```python
from build123d import *

# Parameters (mm, degrees)
SKETCH2_R              = 24.13
SKETCH2_R_2            = 20.447
BASE_DEPTH             = 304.8
SNAP_RING_GROOVE_START = -6.35
SKETCH3_R              = 21.9075
SKETCH3_R_2            = 20.447
SNAP_RING_GROOVE_DEPTH = 1.7272


with BuildPart() as part:
    # Sketch2 → base (new body)
    with BuildSketch(Plane(origin=(0, 0, 0), x_dir=(0, 1, 0), z_dir=(0, 0, 1))):
        with Locations(Location((0, 0, 0), (0, 0, 90))):
            Circle(SKETCH2_R)
        with Locations(Location((0, 0, 0), (0, 0, 90))):
            Circle(SKETCH2_R_2, mode=Mode.SUBTRACT)
    extrude(amount=BASE_DEPTH)

    # Sketch3 → snap_ring_groove (cut)
    with BuildSketch(Plane(origin=(0, 0, 0), x_dir=(1, 0, 0), z_dir=(0, 0, -1)).offset(SNAP_RING_GROOVE_START)):
        with Locations(Location((0, 0, 0), (0, 0, 180))):
            Circle(SKETCH3_R)
        with Locations(Location((0, 0, 0), (0, 0, 180))):
            Circle(SKETCH3_R_2, mode=Mode.SUBTRACT)
    extrude(amount=-SNAP_RING_GROOVE_DEPTH, mode=Mode.SUBTRACT)


solid = part.part
```
Part model, mm, in its own coordinate system. A direction names the side the tool comes from. Coordinates: 2 decimals unless noted, no trailing zeros. Write each loop counter-clockwise with the first axis right and the second up, starting at its lowest first coordinate (ties: lowest second). Pieces come first, ordered by that corner, then holes.
Item 1: Slice it at A-A (x = 0). Write the cut outline in (y, z).
Item 2: Pin check, flat tips, straight feed: pin 1 (10 mm diameter, centred on x = 0, z = 223.5, fed in from +Y); pin 2 (24.5 mm diameter, centred on x = 0, y = 0, fed in from -Z); pin 3 (3 mm diameter, centred on x = 13, z = 257, fed in from -Y); pin 4 (12 mm diameter, centred on y = 10, z = 267, fed in from -X). Stop position of each tip, or through.
Item 3: Probe line 1 (Z direction, x = 4, y = 20.5); line 2 (Y direction, x = 0, z = 7.5); line 3 (Y direction, x = 0, z = 90.5). List the from-to ranges inside material, lowest first.
Item 4: Slice it at C-C (z = 184.5). Write the cut outline in (x, y), and give its area (3 significant figures).
Item 5: Which spindle directions (+Z, -Z, +X, -X, +Y, -Y) get a long thin tool onto all of the face, cutting with end or side? Do faces 1 (the face through (4.749, -21.387, 7.202)), 2 (the face through (20, -5, 0)). Say none if no direction does.
Item 6: Mould opens along Z. For faces 3 (the face through (20, -5, 304.8)), 4 (the face through (16.226, 12.442, 154.362)), 5 (the face through (-15, -15, 8.077)), 6 (the face through (-15, -15, 6.35)) say: released by +Z, released by -Z, zero draft, split by the parting line, or undercut.
Results found:
1. outline: (-24.13, 0) - (-20.45, 0) - (-20.45, 6.35) - (-21.91, 6.35) - (-21.91, 8.08) - (-20.45, 8.08) - (-20.45, 304.8) - (-24.13, 304.8) - close; (20.45, 0) - (24.13, 0) - (24.13, 304.8) - (20.45, 304.8) - (20.45, 8.08) - (21.91, 8.08) - (21.91, 6.35) - (20.45, 6.35) - close
2. pin 1: stops at y = 24.13
2. pin 2: passes through
2. pin 3: stops at y = -21.21
2. pin 4: stops at x = -23.8
3. line 1: z = 0 to 6.35, 8.08 to 304.8
3. line 2: y = -24.13 to -21.91, 21.91 to 24.13
3. line 3: y = -24.13 to -20.45, 20.45 to 24.13
4. outline: circle Ø48.26 at (0, 0); hole circle Ø40.89 at (0, 0)
4. area: 516 mm2
5. face 1: none
5. face 2: -Z, +X, -X, +Y, -Y
6. face 3: released by +Z
6. face 4: zero draft
6. face 5: undercut
6. face 6: undercut
